```python
from build123d import *

# Parameters (mm, degrees)
SKETCH3_W           = 12.984343194
SKETCH3_H           = 2.380771229
SKETCH3_W_2         = 4.803091943
SKETCH3_H_2         = 9.313818956
BOSS_EXTRUDE2_DEPTH = 32.27
SKETCH6_W           = 8
SKETCH6_H           = 4.803091943
BOSS_EXTRUDE3_DEPTH = 10
CUT_EXTRUDE2_DEPTH  = 1.25
FILLET1_R           = 3


with BuildPart() as part:
    # Sketch3 → Boss-Extrude2 (new body)
    with BuildSketch(Plane(origin=(0, 0, 0), x_dir=(0, 0, -1), z_dir=(1, 0, 0))):
        with Locations((0.543022473, -13.14020457)):
            Rectangle(SKETCH3_W, SKETCH3_H)
        with Locations((0.543022474, -8.974909478)):
            Rectangle(SKETCH3_W_2, SKETCH3_H_2)
    boss_extrude2 = extrude(amount=BOSS_EXTRUDE2_DEPTH)

    # Sketch6 → Boss-Extrude3 (add)
    with BuildSketch(Plane(origin=(0, -4.318, 0), x_dir=(1, 0, 0), z_dir=(0, 1, 0))):
        with Locations((11.27, 0.543022474)):
            Rectangle(SKETCH6_W, SKETCH6_H)
    boss_extrude3 = extrude(amount=BOSS_EXTRUDE3_DEPTH)

    # Sketch7 → Cut-Extrude2 (cut, symmetric)
    with BuildSketch(Plane.XY.offset(-0.543022473)):
        with BuildLine():
            Line((11.27, 5.682), (8.27, 5.682))
            Line((8.27, 5.682), (8.27, -0.520355546))
            ThreePointArc((8.27, -0.520355546), (9.148679656, -2.64167589), (11.27, -3.520355546))
            Line((11.27, -3.520355546), (15.27, -3.520355546))
            Line((15.27, -3.520355546), (15.27, -0.520355546))
            Line((15.27, -0.520355546), (11.27, -0.520355546))
            Line((11.27, -0.520355546), (11.27, 5.682))
        make_face()
    cut_extrude2 = extrude(amount=CUT_EXTRUDE2_DEPTH, both=True, mode=Mode.SUBTRACT)

    # Fillet1
    fillet1_edges = [part.edges().sort_by_distance(p)[0] for p in [
        (11.27, -0.520355546, -0.543022473),
    ]]
    fillet(fillet1_edges, radius=FILLET1_R)

    # Mirror2: Boss-Extrude2, Boss-Extrude3, Cut-Extrude2 across plane
    add(boss_extrude2.mirror(Plane.ZY.offset(-32.27)))
    add(boss_extrude3.mirror(Plane.ZY.offset(-32.27)))
    add(cut_extrude2.mirror(Plane.ZY.offset(-32.27)), mode=Mode.SUBTRACT)


solid = part.part
```
Could you check a few things on this model? Use its own coordinates, in mm. A direction names the side the tool comes from. Round coordinates to 2 decimals unless told otherwise and drop trailing zeros. Write each loop counter-clockwise with the first axis right and the second up, starting at its lowest first coordinate (ties: lowest second). Pieces come first, ordered by that corner, then holes.
(1) If I drill on probe 1 along Z at (x, y) = (10, -1.5); probe 2 along X at (y, z) = (-2, -2.75); probe 3 along Z at (x, y) = (60, -5.5), over which ranges is the centre line in solid material (lowest first)?
Findings below:
probe 1: z = -2.94 to -1.79, 0.71 to 1.86
probe 2: x = 7.27 to 15.27, 49.27 to 57.27
probe 3: z = -2.94 to 1.86
(2) Suppose I cut it at C-C on x = 50. Write out the boundary of the cut face in (y, z), and give its area (3 significant figures).
Findings below:
outline: (-14.33, -7.04) - (-11.95, -7.04) - (-11.95, -2.94) - (5.68, -2.94) - (5.68, 1.86) - (-11.95, 1.86) - (-11.95, 5.95) - (-14.33, 5.95) - close; hole (-3.52, -1.79) - (-0.52, -1.79) - (-0.52, 0.71) - (-3.52, 0.71) - close
area: 108 mm2
(3) Which directions (+Z, -Z, +X, -X, +Y, -Y) give clear straight access to the entire face, cutting with the end or side of a thin tool? Please do faces 5 (the face through (15.27, 1, -1)), 6 (the face through (55.41, -2.62, -0.53)), 7 (the face through (4, -4.318, -1)), 8 (the face through (57.27, 1, -1)).
Findings below:
face 5: +Z, -Z, +Y
face 6: +Y
face 7: +Z, -Z, -X, +Y
face 8: +Z, -Z, +X, +Y
(4) For pin 1 (5.5 mm diameter, centred on y = 3, z = 0, fed in from +X); pin 2 (2 mm diameter, centred on x = 37, z = 3, fed in from +Y); pin 3 (4 mm diameter, centred on x = 39.5, z = 3, fed in from +Y); pin 4 (2 mm diameter, centred on y = -6.5, z = -5, fed in from -X), each with a flat end and sliding along its axis, tell me the tip position at first contact or that it passes through.
Findings below:
pin 1: stops at x = 57.27
pin 2: stops at y = -11.95
pin 3: stops at y = -4.32
pin 4: passes through
(5) Suppose I cut it at D-D on x = 38. Write out the boundary of the cut face in (y, z), and give its area (3 significant figures).
Findings below:
outline: (-14.33, -7.04) - (-11.95, -7.04) - (-11.95, -2.94) - (-4.32, -2.94) - (-4.32, 1.86) - (-11.95, 1.86) - (-11.95, 5.95) - (-14.33, 5.95) - close
area: 67.6 mm2
(6) Suppose I cut it at B-B on z = -0.5. Write out the boundary of the cut face in (x, y), and give its area (3 significant figures).
Findings below:
outline: (0, -14.33) - (64.54, -14.33) - (64.54, -4.32) - (57.27, -4.32) - (57.27, 5.68) - (56.27, 5.68) - (56.27, -0.52) arc R3 cw to (53.27, -3.52) - (49.27, -3.52) - (49.27, -4.32) - (15.27, -4.32) - (15.27, -3.52) - (11.27, -3.52) arc R3 cw to (8.27, -0.52) - (8.27, 5.68) - (7.27, 5.68) - (7.27, -4.32) - (0, -4.32) - close; (11.27, 2.48) arc R3 ccw to (14.27, -0.52) - (15.27, -0.52) - (15.27, 5.68) - (11.27, 5.68) - close; (49.27, -0.52) - (53.27, -0.52) - (53.27, 5.68) - (49.27, 5.68) - close
area: 729 mm2
(7) Suppose I cut it at A-A on y = 4.5. Write out the boundary of the cut face in (x, z), and give its area (3 significant figures).
Findings below:
outline: (7.27, -2.94) - (15.27, -2.94) - (15.27, 1.86) - (7.27, 1.86) - close; (49.27, -2.94) - (57.27, -2.94) - (57.27, 1.86) - (49.27, 1.86) - close; hole (8.27, -1.79) - (11.27, -1.79) - (11.27, 0.71) - (8.27, 0.71) - close; hole (53.27, -1.79) - (56.27, -1.79) - (56.27, 0.71) - (53.27, 0.71) - close
area: 61.8 mm2
(8) Thinking about a two-plate mould opening in X: for faces 1 (the face through (0, -10, 0)), 2 (the face through (53.27, 3, -1)), 3 (the face through (49.27, 1, -1)), 4 (the face through (12, 5.682, -1)), which applies, +X half, -X half, draft (parallel to the pull), parting line (faces both ways), or undercut?
Findings below:
face 1: -X half
face 2: undercut
face 3: undercut
face 4: draft
